Here's how the part is built. I have some questions about the finished solid (model axes, mm). Face numbers are marked on the shaded views. A direction names the side the tool comes from. Round coordinates to 2 decimals unless told otherwise and drop trailing zeros. Write each loop counter-clockwise with the first axis right and the second up, starting at its lowest first coordinate (ties: lowest second). Pieces come first, ordered by that corner, then holes. Notation, with made-up numbers: (-13.75, -1.75) - (17.25, -1.75) arc R17 cw to (17.25, 30.25) - close; hole circle Ø1 at (-23.75, 59.25). An arc over 180 degrees is marked (long way). One line per item, written item: value. Start each with the question number.
Item 1: Imagine slicing it at D-D, the plane x = -2. Please give me the cut outline in (y, z), then the cut area to 3 significant figures.
Item 2: If I drill on line 1 (Y direction, x = 0, z = 0.25); line 2 (Z direction, x = -1, y = -1); line 3 (Y direction, x = 0.25, z = 1.95), over which ranges is the centre line in solid material (lowest first)?
Item 3: Thinking about a two-plate mould opening in Z: for the marked faces 4, 5 and 6, which applies, released by +Z, released by -Z, zero draft, split by the parting line, or undercut?
Item 4: Imagine slicing it at C-C, the plane y = 2.25. Please give me the cut outline in (x, z).
Item 5: Imagine slicing it at A-A, the plane x = 0. Please give me the cut outline in (y, z).
Item 6: Imagine slicing it at B-B, the plane z = 1.25. Please give me the cut outline in (x, y) (3 decimals), then the cut area to 3 significant figures.
Item 7: For P1, Ø0.8, axis at y = -5.5, z = 1.5, coming from the -X side; P2, Ø0.8, axis at x = -1.5, z = 2, coming from the -Y side, each with a flat end and sliding along its axis, tell me the tip position at first contact or that it passes through.
Item 8: For the marked faces 1, 2 and 3, which set-ups out of +Z, -Z, +X, -X, +Y, -Y let a thin tool reach every point of the face, with its end or its side?
```python
from build123d import *

# Parameters (mm, degrees)
SKETCH1_R           = 1.375
BOSS_EXTRUDE1_DEPTH = 3
CUT_EXTRUDE1_DEPTH  = 0.98


with BuildPart() as part:
    # Sketch1 → Boss-Extrude1 (new body)
    with BuildSketch(Plane.XY):
        with BuildLine():
            Line((-1, -5), (-1, -6))
            Line((-1, -6), (1, -6))
            Line((1, -6), (1, -5))
            Line((1, -5), (3.5, -5))
            Line((3.5, -5), (3.5, 4))
            ThreePointArc((3.5, 4), (3.207106781, 4.707106781), (2.5, 5))
            Line((2.5, 5), (-2.5, 5))
            ThreePointArc((-2.5, 5), (-3.207106781, 4.707106781), (-3.5, 4))
            Line((-3.5, 4), (-3.5, -5))
            Line((-3.5, -5), (-1, -5))
        make_face()
        with Locations((0, 1.325)):
            Circle(SKETCH1_R, mode=Mode.SUBTRACT)
    extrude(amount=BOSS_EXTRUDE1_DEPTH)

    # Sketch2 → Cut-Extrude1 (cut, symmetric)
    with BuildSketch(Plane.XY.offset(1.5)):
        Polygon((3.031088913, 1.325), (1.515544457, 3.95), (-1.515544457, 3.95), (-3.031088913, 1.325), (-1.515544457, -1.3), (1.515544457, -1.3), align=None)
    extrude(amount=CUT_EXTRUDE1_DEPTH, both=True, mode=Mode.SUBTRACT)


solid = part.part
```
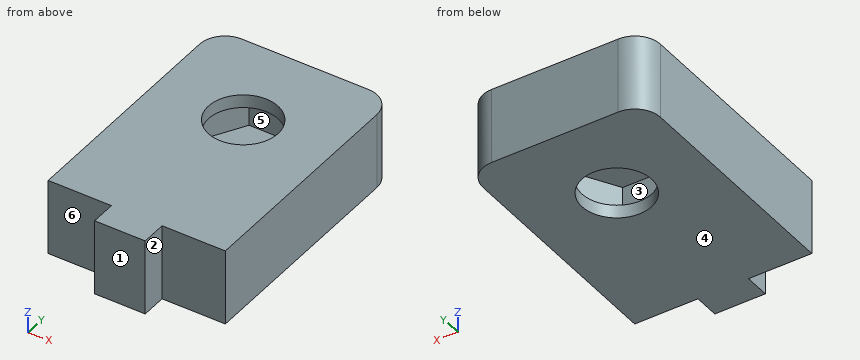
Values follow:
1. outline: (-5, 0) - (5, 0) - (5, 3) - (-5, 3) - close; hole (-0.46, 0.52) - (3.11, 0.52) - (3.11, 2.48) - (-0.46, 2.48) - close
1. area: 23.0 mm^2
2. line 1: y = -6 to -0.05, 2.7 to 5
2. line 2: z = 0 to 0.52, 2.48 to 3
2. line 3: y = -6 to -1.3, 3.95 to 5
3. face 4: released by -Z
3. face 5: undercut
3. face 6: zero draft
4. outline: (-3.5, 0) - (-1.02, 0) - (-1.02, 0.52) - (-2.5, 0.52) - (-2.5, 2.48) - (-1.02, 2.48) - (-1.02, 3) - (-3.5, 3) - close; (1.02, 0) - (3.5, 0) - (3.5, 3) - (1.02, 3) - (1.02, 2.48) - (2.5, 2.48) - (2.5, 0.52) - (1.02, 0.52) - close
5. outline: (-6, 0) - (-0.05, 0) - (-0.05, 0.52) - (-1.3, 0.52) - (-1.3, 2.48) - (-0.05, 2.48) - (-0.05, 3) - (-6, 3) - close; (2.7, 0) - (5, 0) - (5, 3) - (2.7, 3) - (2.7, 2.48) - (3.95, 2.48) - (3.95, 0.52) - (2.7, 0.52) - close
6. outline: (-3.5, -5) - (-1, -5) - (-1, -6) - (1, -6) - (1, -5) - (3.5, -5) - (3.5, 4) arc R1 ccw to (2.5, 5) - (-2.5, 5) arc R1 ccw to (-3.5, 4) - close; hole (-3.031, 1.325) - (-1.516, -1.3) - (1.516, -1.3) - (3.031, 1.325) - (1.516, 3.95) - (-1.516, 3.95) - close
6. area: 47.7 mm^2
7. P1: stops at x = -1
7. P2: stops at y = -5
8. face 1: +Z, -Z, +X, -X, -Y
8. face 2: +Z, -Z, +X, -Y
8. face 3: none
